Design review of the part shown in the three views and the two pictorial views. Dimensions are in mm from the part's minimum x, y and z. A direction names the side the tool comes from. Coordinates: 2 decimals unless noted, no trailing zeros. Write each loop counter-clockwise with the first axis right and the second up, starting at its lowest first coordinate (ties: lowest second). Pieces come first, ordered by that corner, then holes. Notation, with made-up numbers: (55.25, 14) - (62.25, 14) arc R17 cw to (62.25, 46) - close; hole circle Ø1 at (1.25, 80). An arc over 180 degrees is marked (long way). Write each question's results on one line, items separated by ' | '.
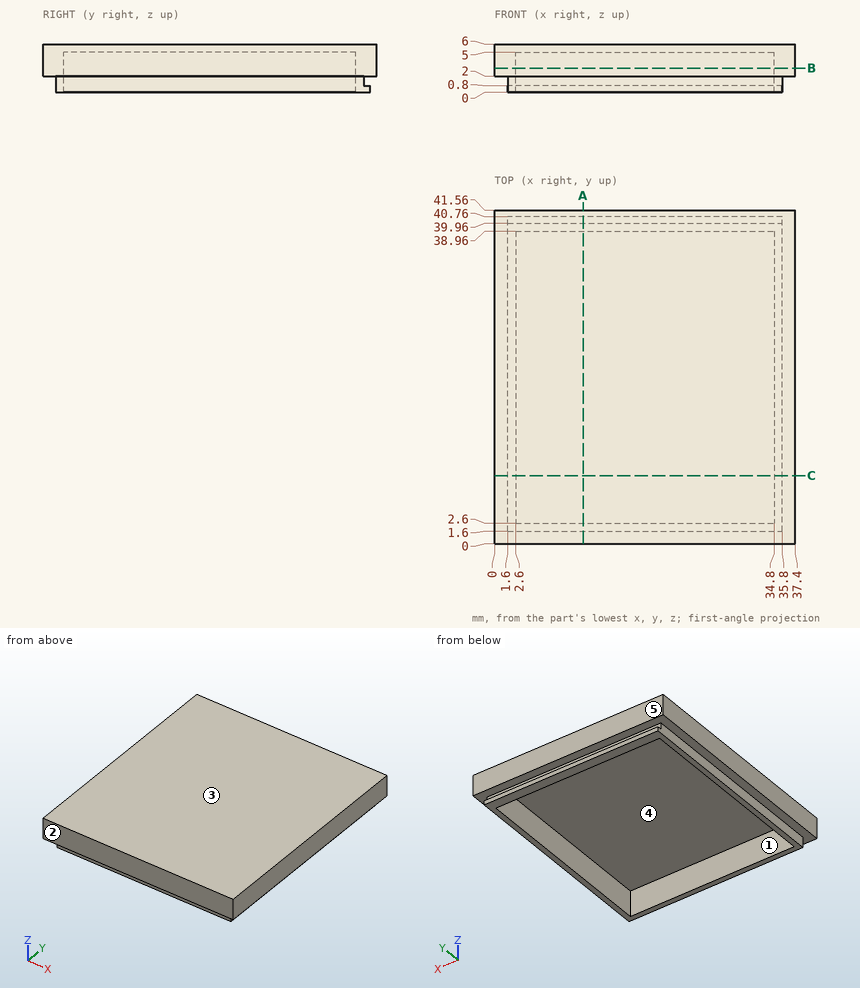
Q1. For pin 1 (18.5 mm diameter, centred on x = 23.5, y = 28.5, fed in from -Z); pin 2 (1 mm diameter, centred on x = 20.5, z = 1, fed in from -Y); pin 3 (1.3 mm diameter, centred on x = 26, z = 1, fed in from +Y), all flat-tipped, find the tip position at first contact; note any pin that passes through.
Results found:
pin 1: z = 5 | pin 2: y = 1.6 | pin 3: y = 40.76
Q2. For the marked faces 1 and 2, list the 3-axis set-ups (+Z, -Z, +X, -X, +Y, -Y) from which the entire face can be reached by the end or side of a thin tool; tool diameter is ignored.
Results found:
face 1: -Z | face 2: +Z, -Z, +X, -X, -Y
Q3. Take a section at C-C on y = 8.5. State the section outline as (x, z) points, plus the area to 3 significant figures.
Results found:
outline: (0, 2) - (1.6, 2) - (1.6, 0) - (2.6, 0) - (2.6, 5) - (34.8, 5) - (34.8, 0) - (35.8, 0) - (35.8, 2) - (37.4, 2) - (37.4, 6) - (0, 6) - close | area: 57.0 mm2
Q4. Take a section at B-B on z = 3. State the section outline as (x, y) points.
Results found:
outline: (0, 0) - (37.4, 0) - (37.4, 41.56) - (0, 41.56) - close; hole (2.6, 2.6) - (34.8, 2.6) - (34.8, 38.96) - (2.6, 38.96) - close
Q5. Mouldability with a two-part tool opening along Y and no side actions: class the marked faces 3, 4 and 5 as pulls with the +Y half, pulls with the -Y half, needs draft (parallel to the pull), parting line crosses it, or undercut.
Results found:
face 3: needs draft | face 4: undercut | face 5: pulls with the +Y half
Q6. Wall thickness on line 1 along X through (y, z) = (21.5, 1); line 2 along Y through (x, z) = (9, 1.75); line 3 along X through (y, z) = (25.5, 4.5): over which ranges is each line inside the solid? List them lowest first. Write a range as from..to.
Results found:
line 1: 1.6..2.6, 34.8..35.8 | line 2: 1.6..2.6, 38.96..39.96 | line 3: 0..2.6, 34.8..37.4
Q7. Take a section at A-A on x = 11. State the section outline as (y, z) points, plus the area to 3 significant figures.
Results found:
outline: (0, 2) - (1.6, 2) - (1.6, 0) - (2.6, 0) - (2.6, 5) - (38.96, 5) - (38.96, 0) - (40.76, 0) - (40.76, 0.8) - (39.96, 0.8) - (39.96, 2) - (41.56, 2) - (41.56, 6) - (0, 6) - close | area: 61.8 mm2
